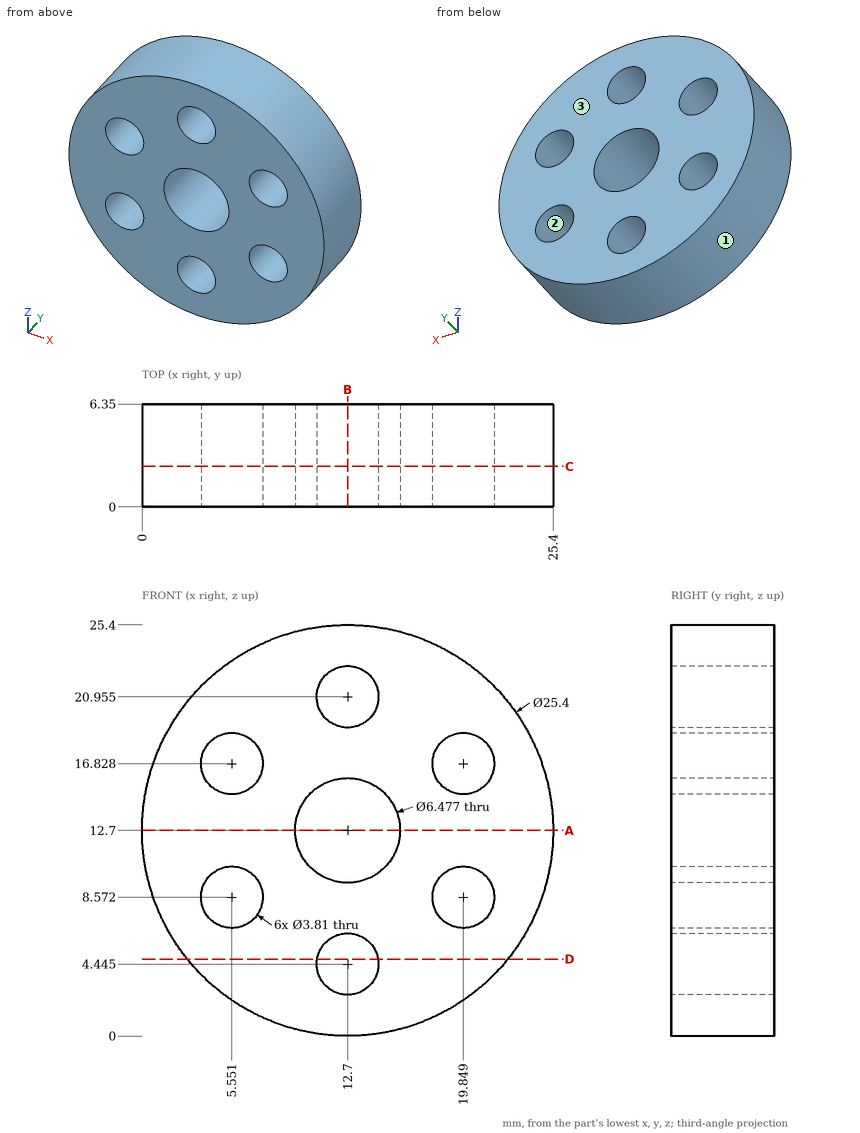
Print and shaded views of the part. All mm, measured from the part's lowest x, y and z. Round coordinates to 2 decimals unless told otherwise and drop trailing zeros. Write each loop counter-clockwise with the first axis right and the second up, starting at its lowest first coordinate (ties: lowest second). Pieces come first, ordered by that corner, then holes. Notation, with made-up numbers: M -1,19.25 L 24,19.25 A24 cw 24,54.25 Z; hole C 85.25,3.5 d7. An arc over 180 degrees is marked long. One line per question, with ' | ' between items.
(1) Saw through at A-A on z = 12.7. Write the cut outline in (x, y).
Answer key:
outline: M 0,0 L 9.46,0 L 9.46,6.35 L 0,6.35 Z; M 15.94,0 L 25.4,0 L 25.4,6.35 L 15.94,6.35 Z
(2) Two-plate mould, pull along X, no slides. Class the marked faces 1, 2 and 3: released by +X, released by -X, zero draft, split by the parting line, or undercut.
Answer key:
face 1: split by the parting line | face 2: undercut | face 3: zero draft
(3) Probe line 1 along Z through (x, y) = (12.75, 1); line 2 along X through (y, z) = (3.25, 8.5) (1 decimal); line 3 along Z through (x, y) = (13.75, 5.5) (1 decimal). List the from-to ranges inside material, lowest first.
Answer key:
line 1: z = 0 to 2.54, 6.35 to 9.46, 15.94 to 19.05, 22.86 to 25.4 | line 2: x = 0.7 to 3.6, 7.5 to 17.9, 21.8 to 24.7 | line 3: z = 0 to 2.9, 6 to 9.6, 15.8 to 19.4, 22.5 to 25.4
(4) Saw through at B-B on x = 12.7. Write the cut outline in (y, z).
Answer key:
outline: M 0,0 L 6.35,0 L 6.35,2.54 L 0,2.54 Z; M 0,6.35 L 6.35,6.35 L 6.35,9.46 L 0,9.46 Z; M 0,15.94 L 6.35,15.94 L 6.35,19.05 L 0,19.05 Z; M 0,22.86 L 6.35,22.86 L 6.35,25.4 L 0,25.4 Z
(5) Saw through at C-C on y = 2.5. Count the separate pieces of the cut face and the enclosed holes in it.
Answer key:
separate pieces: 1 | enclosed holes: 7
(6) Saw through at D-D on z = 4.75. Write the cut outline in (x, y), then the cut area to 3 significant figures.
Answer key:
outline: M 2.8,0 L 10.82,0 L 10.82,6.35 L 2.8,6.35 Z; M 14.58,0 L 22.6,0 L 22.6,6.35 L 14.58,6.35 Z | area: 102 mm^2
(7) Pin check, flat tips, straight feed: pin 1 (3 mm diameter, centred on x = 12.7, z = 20.955, fed in from -Y); pin 2 (3 mm diameter, centred on x = 12, z = 3.5, fed in from +Y). Stop position of each tip, or through.
Answer key:
pin 1: passes through | pin 2: stops at y = 6.35
